Could you check a few things on this model? Use its own coordinates, in mm. A direction names the side the tool comes from. Round coordinates to 2 decimals unless told otherwise and drop trailing zeros. Loops run counter-clockwise (first coordinate to the right, second up) from the corner with the lowest first, then second, coordinate; pieces in that order, holes last. Notation, with made-up numbers: M 42.5,27 L 63.5,27 A22 ccw 63.5,55 Z; hole C 51,45.25 d11. An arc over 180 degrees is marked long. Return JSON: item names as keys, results as strings. Group by question number.
Autodesk Inventor part; units mm, degrees
ref_plane "YZ Plane" through (0, 0, 0) normal (1, 0, 0) x (0, 1, 0)
ref_plane "XZ Plane" through (0, 0, 0) normal (0, 1, 0) x (-1, 0, 0)
ref_plane "XY Plane" through (0, 0, 0) normal (0, 0, 1) x (1, 0, 0)
sketch "Sketch1" plane through (0, 0, 0) normal (0, 0, 1) x (1, 0, 0)
  line L0 (0, 0) -> (14.1421, -14.1421)
  line L1 (0, 0) -> (20, 0) construction
  line L2 (14.1421, -14.1421) -> (15.5563, -12.7279)
  line L3 (15.5563, -12.7279) -> (1.4142, 1.4142)
  line L4 (1.4142, 1.4142) -> (0, 0)
  line L5 (1.4142, 1.4142) -> (15.5563, 1.4142)
  line L6 (14.1421, -14.1421) -> (14.1421, -34.1421)
  line L7 (14.1421, -34.1421) -> (16.1421, -34.1421)
  line L8 (16.1421, -34.1421) -> (16.1421, 1.4142)
  line L9 (16.1421, 1.4142) -> (15.5563, 1.4142)
  dimension "d0" = 20
  dimension "d1" = 45
  dimension "d2" = 2
  dimension "d3" = 20
  dimension "d4" = 20
  dimension "d6" = 2
extrude "Extrusion1" add sketch "Sketch1" along normal blind 27
sketch "Sketch2" plane through (14.1421, -14.1421, 27) normal (-0.7071, -0.7071, 0) x (-0.7071, 0.7071, 0)
  line L0 (20, 27) -> (0, 27)
  line L1 (0, 27) -> (0, 0)
  line L2 (0, 27) -> (10, 27)
  line L3 (10, 27) -> (10, 13.5)
  line L4 (20, 27) -> (20, 0)
  line L5 (10, 13.5) -> (10, 19.5)
  line L6 (10, 19.5) -> (15, 19.5)
  line L7 (15, 19.5) -> (15, 7.5)
  line L8 (15, 7.5) -> (5, 7.5)
  line L9 (5, 7.5) -> (5, 19.5)
  line L10 (5, 19.5) -> (10, 19.5)
  line L11 (10, 13.5) -> (10, 23.5)
  circle A0 centre (10, 23.5) radius 1.5
  circle A1 centre (10, 23.5) radius 3.5
  line L12 (10, 13.5) -> (10, 3.5)
  circle A2 centre (10, 3.5) radius 1.5
  circle A3 centre (10, 3.5) radius 3.5
  dimension "d20" = 10
  dimension "d21" = 6
  dimension "d22" = 5
  dimension "d23" = 12
  dimension "d24" = 10
  dimension "d25" = 10
  dimension "d26" = 3
  dimension "d27" = 7
  dimension "d28" = 10
  dimension "d29" = 3
  dimension "d30" = 7
properties part number "Time of Flight 4.0"
1. I need wall thicknesses on probe 1 along X at (y, z) = (-22, 7.25); probe 2 along Y at (x, z) = (12.75, 25.5); probe 3 along X at (y, z) = (-9.5, 13.25). Which ranges of each line are inside material? Lowest first, please.
2. I'm going to push flat-ended pins straight in: pin 1 Ø4 at (y, z) = (-25, 9.5) entering from -X; pin 2 Ø12 at (y, z) = (-17.5, 17.5) entering from -X; pin 3 Ø8 at (x, y) = (11, -13.5) entering from -Z. Where does each tip first touch, or does it pass through?
3. If we section it at B-B, the plane x = 4.75: Please give me the cut outline in (y, z).
4. On a 3-axis mill with a long thin cutter (end or side, diameter ignored), from which of +Z, -Z, +X, -X, +Y, -Y can I reach the whole of each face in a straight line? I mean faces 1 (the face through (11, -8, 27)), 2 (the face through (14.142, -24, 13)). Say none if no direction works.
5. If we section it at A-A, the plane z = 4.5: Please give me the cut outline in (x, y).
6. If we section it at C-C, the plane y = -7.5: Please give me the cut outline in (x, z), then the cut area to 3 significant figures.
Geometry results:
{
 "1": {"probe 1": "14.14 to 16.14", "probe 2": "-12.75 to 1.41", "probe 3": "9.5 to 16.14"},
 "2": {"pin 1": "x = 14.14", "pin 2": "x = 11.5", "pin 3": "z = 0"},
 "3": {"outline": "M -4.75,0 L 1.41,0 L 1.41,27 L -4.75,27 Z"},
 "4": {"face 1": "+Z, +X, -X, +Y, -Y", "face 2": "+Z, -Z, -X, -Y"},
 "5": {"outline": "M 0,0 L 14.14,-14.14 L 14.14,-34.14 L 16.14,-34.14 L 16.14,1.41 L 1.41,1.41 Z"},
 "6": {"outline": "M 7.5,0 L 16.14,0 L 16.14,27 L 7.5,27 Z", "area": "233 mm^2"}
}
